Autodesk Inventor part; units mm, degrees
ref_plane "YZ Plane" through (0, 0, 0) normal (1, 0, 0) x (0, 1, 0)
ref_plane "XZ Plane" through (0, 0, 0) normal (0, 1, 0) x (-1, 0, 0)
ref_plane "XY Plane" through (0, 0, 0) normal (0, 0, 1) x (1, 0, 0)
sketch "Эскиз1" plane through (0, 0, 0) normal (0, 1, 0) x (-1, 0, 0)
  line L0 (0, 0) -> (0, -96)
  line L1 (0, 0) -> (15, 0)
  line L2 (15, 0) -> (15, 5)
  line L3 (15, 5) -> (39, 5)
  line L4 (39, 5) -> (39, -5)
  line L5 (39, -5) -> (49, -5)
  line L6 (49, -5) -> (49, -15)
  line L7 (49, -15) -> (55, -15)
  line L8 (55, -15) -> (55, -92)
  line L9 (55, -92) -> (50, -92)
  line L10 (50, -92) -> (45, -97)
  line L11 (45, -97) -> (45, -104)
  line L12 (0, 0) -> (-15, 0)
  line L13 (-15, 0) -> (-15, 5)
  line L14 (-15, 5) -> (-39, 5)
  line L15 (-39, 5) -> (-39, -5)
  line L16 (-39, -5) -> (-49, -5)
  line L17 (-49, -5) -> (-49, -15)
  line L18 (-49, -15) -> (-55, -15)
  line L19 (-55, -15) -> (-55, -92)
  line L20 (-55, -92) -> (-50, -92)
  line L21 (-50, -92) -> (-45, -97)
  line L22 (-45, -97) -> (-45, -104)
  line L23 (45, -104) -> (40, -109)
  line L24 (-40, -109) -> (-45, -104)
  line L25 (40, -109) -> (8.5, -109)
  line L26 (8.5, -109) -> (8.5, -96)
  line L27 (8.5, -96) -> (0, -96)
  line L28 (-40, -109) -> (-8.5, -109)
  line L29 (-8.5, -109) -> (-8.5, -96)
  line L30 (-8.5, -96) -> (0, -96)
  point P0 (45, -109)
  point P1 (-45, -109)
  dimension "d0" = 30
  dimension "d1" = 78
  dimension "d2" = 10
  dimension "d3" = 10
  dimension "d4" = 10
  dimension "d5" = 6
  dimension "d6" = 97
  dimension "d7" = 100
  dimension "d8" = 45
  dimension "d10" = 5
  dimension "d11" = 12
  dimension "d26" = 5
  dimension "d27" = 5
  dimension "d28" = 5
  dimension "d29" = 5
  dimension "d30" = 114
  dimension "d31" = 135
  dimension "d32" = 17
  dimension "d33" = 13
extrude "Выдавливание1" add sketch "Эскиз1" along normal blind 4
sketch "Эскиз2" plane through (0, 4, 0) normal (0, 1, 0) x (1, 0, 0)
  line L0 (0, 0) -> (0, 94.8396)
  line L1 (49, 5) -> (49, 15)
  line L2 (39, 5) -> (49, 5)
  line L3 (-39, -5) -> (-15, -5)
  line L4 (55, 15) -> (55, 92)
  line L5 (55, 92) -> (50, 92)
  line L6 (-55, 92) -> (-55, 15)
  line L7 (-55, 15) -> (-49, 15)
  point P0 (-38, 102.8)
  point P1 (38, 102.8)
  point P2 (44, 9.4)
  point P3 (-44, 9.4)
  dimension "d21" = 5
  dimension "d22" = 4.4
  dimension "d24" = 107.8
  dimension "d25" = 76
hole "Отверстие1" at (-38, 4, -102.8) at (38, 4, -102.8) at (44, 4, -9.4) at (-44, 4, -9.4) direction (0, -1, 0) diameter 2.8 end through all
sketch "Эскиз4" plane through (0, 4, 0) normal (0, 1, 0) x (1, 0, 0)
  line L0 (-55, 92) -> (-55, 15)
  line L1 (-55, 88) -> (-25, 88)
  line L2 (-25, 88) -> (-25, 19)
  line L3 (-25, 19) -> (-55, 19)
  line L4 (-55, 19) -> (-55, 88)
  line L5 (-25, 88) -> (-21, 88)
  line L6 (-21, 88) -> (-21, 74)
  line L7 (-21, 74) -> (-25, 74)
  line L8 (-25, 61.5) -> (-21, 61.5)
  line L9 (-21, 61.5) -> (-21, 45.5)
  line L10 (-21, 45.5) -> (-25, 45.5)
  line L11 (-55, 53.5) -> (-25, 53.5) construction
  line L12 (-25, 19) -> (-21, 19)
  line L13 (-21, 19) -> (-21, 33)
  line L14 (-21, 33) -> (-25, 33)
  line L15 (-25, 33) -> (-25, 19)
  line L16 (-50, 92) -> (-55, 92)
  line L17 (-55, 92) -> (-40, 92)
  line L18 (-40, 92) -> (-40, 88)
  line L19 (-40, 88) -> (-55, 88)
  line L20 (-55, 88) -> (-55, 92)
  line L21 (-55, 15) -> (-40, 15)
  line L22 (-40, 15) -> (-40, 19)
  line L23 (-40, 19) -> (-55, 19)
  line L24 (-55, 19) -> (-55, 15)
  line L25 (-21, 23.5) -> (-18, 23.5)
  line L26 (-18, 23.5) -> (-18, 29.5)
  line L27 (-18, 29.5) -> (-21, 29.5)
  line L28 (-21, 29.5) -> (-21, 23.5)
  line L29 (-21, 77.5) -> (-18, 77.5)
  line L30 (-18, 77.5) -> (-18, 83.5)
  line L31 (-18, 83.5) -> (-21, 83.5)
  line L32 (-21, 83.5) -> (-21, 77.5)
  point P0 (0, 0)
  point P1 (-21, 53.5)
  point P2 (-18, 80.5)
  point P3 (-18, 26.5)
  dimension "d48" = 30
  dimension "d50" = 14
  dimension "d51" = 16
  dimension "d52" = 4
  dimension "d55" = 4
  dimension "d56" = 15
  dimension "d57" = 54
  dimension "d58" = 6
  dimension "d59" = 3
extrude "Выдавливание2" cut sketch "Эскиз4" against normal through all
sketch "Эскиз5" plane through (0, 4, 0) normal (0, 1, 0) x (1, 0, 0)
  line L0 (55, 15) -> (55, 92)
  line L1 (15, -5) -> (39, -5)
  point P0 (0, 0)
  point P1 (-13.3, 12)
  point P2 (35, 12)
  point P3 (35, 94.6)
  point P4 (-13.3, 87.1)
  point P5 (2.1, 63.6)
  point P6 (30.1, 63.6)
  dimension "d67" = 48.3
  dimension "d68" = 82.6
  dimension "d69" = 75.1
  dimension "d70" = 28
  dimension "d71" = 4.9
  dimension "d72" = 20
  dimension "d73" = 17
  dimension "d74" = 51.6
hole "Отверстие2" at (-13.3, 4, -12) at (35, 4, -12) at (35, 4, -94.6) at (-13.3, 4, -87.1) at (2.1, 4, -63.6) at (30.1, 4, -63.6) direction (0, -1, 0) diameter 3 end through all
properties part number "ElectronicPlate"
Could you check a few things on this model? Use its own coordinates, in mm. A direction names the side the tool comes from. Round coordinates to 2 decimals unless told otherwise and drop trailing zeros. Order: outer loops, then holes, each group sorted by start corner. A loop starts at its lowest first (then second) coordinate and runs counter-clockwise, first axis right, second up.
Q1. Please list where these lines run through material, in increasing order: probe 1 along X at (y, z) = (1, -102.8); probe 2 along Z at (x, y) = (35, 2.4); probe 3 along X at (y, z) = (0.9, -12).
Geometry says:
probe 1: x = -45 to -39.4, -36.6 to -8.5, 8.5 to 36.6, 39.4 to 45
probe 2: z = -109 to -96.1, -93.1 to -13.5, -10.5 to 5
probe 3: x = -49 to -14.8, -11.8 to 33.5, 36.5 to 49
Q2. Imagine slicing it at C-C, the plane z = -17.5. List the corners of the cut face in (x, y) for me.
Geometry says:
outline: (-40, 0) - (55, 0) - (55, 4) - (-40, 4) - close
Q3. Thinking about a two-plate mould opening in X: for faces 5 (the face through (2.03, 1.97, -65.1)), 6 (the face through (55, 2, -53)), 7 (the face through (-23, 2, -45.5)), 8 (the face through (-45, 2, -100)), which applies, released by +X, released by -X, zero draft, split by the parting line, or undercut?
Geometry says:
face 5: undercut
face 6: released by +X
face 7: zero draft
face 8: released by -X
Q4. Which directions (+Z, -Z, +X, -X, +Y, -Y) give clear straight access to the entire face, cutting with the end or side of a thin tool? Please do faces 1 (the face through (8.5, 2, -103)), 2 (the face through (-44, 2, -5)), 3 (the face through (39, 2, 0)), 4 (the face through (-20, 2, -77.5)).
Geometry says:
face 1: -Z, +Y, -Y
face 2: +Z, -X, +Y, -Y
face 3: +Z, +X, +Y, -Y
face 4: -X, +Y, -Y
Q5. Imagine slicing it at A-A, the plane z = -63.6. List the corners of the cut face in (x, y) for me.
Geometry says:
outline: (-25, 0) - (0.6, 0) - (0.6, 4) - (-25, 4) - close; (3.6, 0) - (28.6, 0) - (28.6, 4) - (3.6, 4) - close; (31.6, 0) - (55, 0) - (55, 4) - (31.6, 4) - close
Q6. Imagine slicing it at B-B, the plane x = 35. List the corners of the cut face in (y, z) for me, then the cut area to 3 significant figures.
Geometry says:
outline: (0, -109) - (4, -109) - (4, -96.1) - (0, -96.1) - close; (0, -93.1) - (4, -93.1) - (4, -13.5) - (0, -13.5) - close; (0, -10.5) - (4, -10.5) - (4, 5) - (0, 5) - close
area: 432 mm2
Q7. Imagine slicing it at D-D, the plane z = -41.5. List the corners of the cut face in (x, y) for me.
Geometry says:
outline: (-25, 0) - (55, 0) - (55, 4) - (-25, 4) - close
Q8. I'm going to push flat-ended pins straight in: P1, Ø2, axis at y = 2, z = -100.5, coming from the -X side; P2, Ø2, axis at x = 41.5, y = 1.5, coming from the +Z side. Where does each tip first touch, or does it pass through?
Geometry says:
P1: stops at x = -45
P2: stops at z = -5
